from build123d import *

# Parameters (mm, degrees)
BOSS_EXTRUDE1_DEPTH = 180
SKETCH2_R           = 12.5
CUT_EXTRUDE1_DEPTH  = 191.91883092


with BuildPart() as part:
    # Sketch1 → Boss-Extrude1 (new body)
    with BuildSketch(Plane(origin=(0, 0, 0), x_dir=(1, 0, 0), z_dir=(0, 1, 0))):
        with BuildLine():
            Line((-45, 0), (-42.5, 0))
            ThreePointArc((-42.5, 0), (0, -42.5), (42.5, 0))
            Line((42.5, 0), (45, 0))
            ThreePointArc((45, 0), (0, -45), (-45, 0))
        make_face()
    extrude(amount=BOSS_EXTRUDE1_DEPTH)

    # Sketch2 → Cut-Extrude1 (cut, through all)
    with BuildSketch(Plane.XY):
        with Locations(Location((0, 135, 0), (0, 0, 180))):
            Circle(SKETCH2_R)
    extrude(amount=CUT_EXTRUDE1_DEPTH, mode=Mode.SUBTRACT)


solid = part.part
Could you check a few things on this model? Use its own coordinates, in mm. Give positions to 0.01 mm unless a question says otherwise; leave off trailing zeros. Write each loop counter-clockwise with the first axis right and the second up, starting at its lowest first coordinate (ties: lowest second). Pieces come first, ordered by that corner, then holes. Notation, with made-up numbers: (8.5, -15) - (41.5, -15) arc R22 ccw to (41.5, 3) - close; hole circle Ø4 at (83, 30.5). An arc over 180 degrees is marked (long way). Use CSV: the item, a comma, the result in double quotes. Start each with the question number.
Item 1: I want a section at C-C, the plane y = 33. Please give me the cut outline in (x, z).
Item 2: If I drill on line 1 along X through (y, z) = (60, 6); line 2 along X through (y, z) = (82.5, 34); line 3 along Z through (x, y) = (-38, 99.5), over which ranges is the centre line in solid material (lowest first)?
Item 3: I want a section at D-D, the plane x = 37.5. Please give me the cut outline in (y, z), then the cut area to 3 significant figures.
Item 4: I want a section at B-B, the plane y = 135. Please give me the cut outline in (x, z).
Item 5: If we mould it in two halves opening along X, with no side actions, what happens to faces 1 (the face through (-6.5, 0, 42.4)), 2 (the face through (-11.923, 131.245, 42.793)), 3 (the face through (0.99, 88.74, 44.99))? For each: pulls with the +X half, pulls with the -X half, needs draft (parallel to the pull), parting line crosses it, or undercut.
Item 6: I'm going to push flat-ended pins straight in: pin 1 (3 mm diameter, centred on y = 116, z = 22.5, fed in from -X); pin 2 (8 mm diameter, centred on x = -12, y = 139, fed in from -Z); pin 3 (4 mm diameter, centred on y = 104.5, z = 27, fed in from +X); pin 4 (12 mm diameter, centred on x = -2, y = 81, fed in from +Z). Where does each tip first touch, or does it pass through?
Item 7: I want a section at A-A, the plane x = 0. Please give me the cut outline in (y, z), then the cut area to 4 significant figures.
Findings:
1,outline,"(-45, 0) - (-42.5, 0) arc R42.5 cw to (42.5, 0) - (45, 0) arc R45 ccw to start"
2,line 1,"x = -44.6 to -42.07, 42.07 to 44.6"
2,line 2,"x = -29.48 to -25.5, 25.5 to 29.48"
2,line 3,"z = 19.03 to 24.1"
3,outline,"(0, 20) - (180, 20) - (180, 24.87) - (0, 24.87) - close"
3,area,"877 mm2"
4,outline,"(-45, 0) - (-42.5, 0) arc R42.5 cw to (-12.5, 40.62) - (-12.5, 43.23) arc R45 ccw to start; (12.5, 40.62) arc R42.5 cw to (42.5, 0) - (45, 0) arc R45 ccw to (12.5, 43.23) - close"
5,face 1,"needs draft"
5,face 2,"undercut"
5,face 3,"parting line crosses it"
6,pin 1,"stops at x = -39.8"
6,pin 2,"stops at z = 39.37"
6,pin 3,"stops at x = 37.42"
6,pin 4,"stops at z = 45"
7,outline,"(0, 42.5) - (122.5, 42.5) - (122.5, 45) - (0, 45) - close; (147.5, 42.5) - (180, 42.5) - (180, 45) - (147.5, 45) - close"
7,area,"387.5 mm2"
